Work out the finished part from the listing and answer in its coordinate system (mm). Round coordinates to 2 decimals unless told otherwise and drop trailing zeros. Write each loop counter-clockwise with the first axis right and the second up, starting at its lowest first coordinate (ties: lowest second). Pieces come first, ordered by that corner, then holes. Notation, with made-up numbers: (74, -13.5) -> (126, -13.5) arc R11 cw to (126, 5.5) -> close; hole circle Ø4 at (35.5, 53). An arc over 180 degrees is marked (long way). Answer as a JSON object with one key per item and string values. Group by question number.
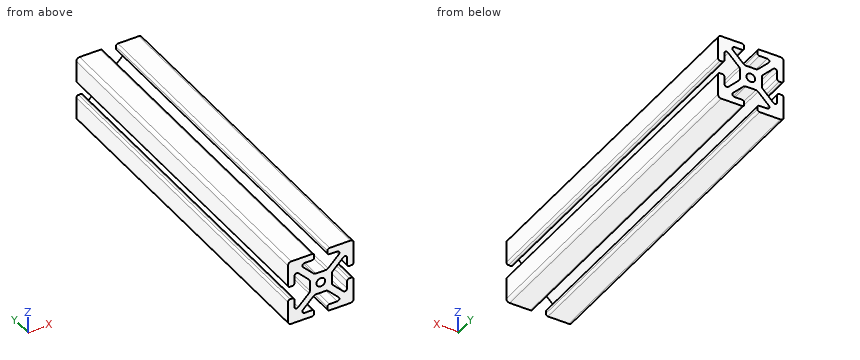
from build123d import *

# Parameters (mm, degrees)
F0_R     = 2
F1_DEPTH = 160


with BuildPart() as f1:
    # F0 (on Front) → F1 (new body)
    with BuildSketch(Plane.XZ):
        with BuildLine():
            ThreePointArc((15, 13.5), (14.56066, 14.56066), (13.5, 15))
            Line((13.5, 15), (4, 15))
            ThreePointArc((4, 15), (3.292893, 14.707107), (3, 14))
            Line((3, 14), (3, 13))
            ThreePointArc((3, 13), (3.292893, 12.292893), (4, 12))
            Line((4, 12), (7.464466, 12))
            ThreePointArc((7.464466, 12), (8.388346, 11.382683), (8.171573, 10.292893))
            Line((8.171573, 10.292893), (3.318019, 5.43934))
            ThreePointArc((3.318019, 5.43934), (2.831384, 5.114181), (2.257359, 5))
            Line((2.257359, 5), (-2.257359, 5))
            ThreePointArc((-2.257359, 5), (-2.831384, 5.114181), (-3.318019, 5.43934))
            Line((-3.318019, 5.43934), (-8.171573, 10.292893))
            ThreePointArc((-8.171573, 10.292893), (-8.388346, 11.382683), (-7.464466, 12))
            Line((-7.464466, 12), (-4, 12))
            ThreePointArc((-4, 12), (-3.292893, 12.292893), (-3, 13))
            Line((-3, 13), (-3, 14))
            ThreePointArc((-3, 14), (-3.292893, 14.707107), (-4, 15))
            Line((-4, 15), (-13.5, 15))
            ThreePointArc((-13.5, 15), (-14.56066, 14.56066), (-15, 13.5))
            Line((-15, 13.5), (-15, 4))
            ThreePointArc((-15, 4), (-14.707107, 3.292893), (-14, 3))
            Line((-14, 3), (-13, 3))
            ThreePointArc((-13, 3), (-12.292893, 3.292893), (-12, 4))
            Line((-12, 4), (-12, 7.464466))
            ThreePointArc((-12, 7.464466), (-11.382683, 8.388346), (-10.292893, 8.171573))
            Line((-10.292893, 8.171573), (-5.43934, 3.318019))
            ThreePointArc((-5.43934, 3.318019), (-5.114181, 2.831384), (-5, 2.257359))
            Line((-5, 2.257359), (-5, -2.257359))
            ThreePointArc((-5, -2.257359), (-5.114181, -2.831384), (-5.43934, -3.318019))
            Line((-5.43934, -3.318019), (-10.292893, -8.171573))
            ThreePointArc((-10.292893, -8.171573), (-11.382683, -8.388346), (-12, -7.464466))
            Line((-12, -7.464466), (-12, -4))
            ThreePointArc((-12, -4), (-12.292893, -3.292893), (-13, -3))
            Line((-13, -3), (-14, -3))
            ThreePointArc((-14, -3), (-14.707107, -3.292893), (-15, -4))
            Line((-15, -4), (-15, -13.5))
            ThreePointArc((-15, -13.5), (-14.56066, -14.56066), (-13.5, -15))
            Line((-13.5, -15), (-4, -15))
            ThreePointArc((-4, -15), (-3.292893, -14.707107), (-3, -14))
            Line((-3, -14), (-3, -13))
            ThreePointArc((-3, -13), (-3.292893, -12.292893), (-4, -12))
            Line((-4, -12), (-7.464466, -12))
            ThreePointArc((-7.464466, -12), (-8.388346, -11.382683), (-8.171573, -10.292893))
            Line((-8.171573, -10.292893), (-3.318019, -5.43934))
            ThreePointArc((-3.318019, -5.43934), (-2.831384, -5.114181), (-2.257359, -5))
            Line((-2.257359, -5), (2.257359, -5))
            ThreePointArc((2.257359, -5), (2.831384, -5.114181), (3.318019, -5.43934))
            Line((3.318019, -5.43934), (8.171573, -10.292893))
            ThreePointArc((8.171573, -10.292893), (8.388346, -11.382683), (7.464466, -12))
            Line((7.464466, -12), (4, -12))
            ThreePointArc((4, -12), (3.292893, -12.292893), (3, -13))
            Line((3, -13), (3, -14))
            ThreePointArc((3, -14), (3.292893, -14.707107), (4, -15))
            Line((4, -15), (13.5, -15))
            ThreePointArc((13.5, -15), (14.56066, -14.56066), (15, -13.5))
            Line((15, -13.5), (15, -4))
            ThreePointArc((15, -4), (14.707107, -3.292893), (14, -3))
            Line((14, -3), (13, -3))
            ThreePointArc((13, -3), (12.292893, -3.292893), (12, -4))
            Line((12, -4), (12, -7.464466))
            ThreePointArc((12, -7.464466), (11.382683, -8.388346), (10.292893, -8.171573))
            Line((10.292893, -8.171573), (5.43934, -3.318019))
            ThreePointArc((5.43934, -3.318019), (5.114181, -2.831384), (5, -2.257359))
            Line((5, -2.257359), (5, 2.257359))
            ThreePointArc((5, 2.257359), (5.114181, 2.831384), (5.43934, 3.318019))
            Line((5.43934, 3.318019), (10.292893, 8.171573))
            ThreePointArc((10.292893, 8.171573), (11.382683, 8.388346), (12, 7.464466))
            Line((12, 7.464466), (12, 4))
            ThreePointArc((12, 4), (12.292893, 3.292893), (13, 3))
            Line((13, 3), (14, 3))
            ThreePointArc((14, 3), (14.707107, 3.292893), (15, 4))
            Line((15, 4), (15, 13.5))
        make_face()
        Circle(F0_R, mode=Mode.SUBTRACT)
    extrude(amount=-F1_DEPTH)


solid = f1.part
1) A cutting plane is placed at A-A on x = 0. Determine the outline of the cut face in (y, z).
2) Straight lines are drawn through the part: L1, parallel to Z at x = 0, y = 45; L2, parallel to X at y = 98.5, z = 11; L3, parallel to Z at x = 8, y = 41.5. For each, find the intervals that lie inside material, in ascending order.
3) Each of these flat-tipped pins is pushed along its axis until it touches: P1, Ø3.5, axis at y = 67, z = 1, coming from the +X side; P2, Ø3.5, axis at y = 114, z = 0.5, coming from the -X side; P3, Ø1.5, axis at x = -3, y = 90, coming from the +Z side. Where does it stop, or does it pass through?
4) A cutting plane is placed at B-B on z = 0. Determine the outline of the cut face in (x, y), plus the area to 3 significant figures.
Established:
{
 "1": {"outline": "(0, -5) -> (160, -5) -> (160, -2) -> (0, -2) -> close; (0, 2) -> (160, 2) -> (160, 5) -> (0, 5) -> close"},
 "2": {"L1": "z = -5 to -2, 2 to 5", "L2": "x = -15 to -8.46, 8.46 to 15", "L3": "z = -15 to -11.84, -10.12 to -5.88, 5.88 to 10.12, 11.84 to 15"},
 "3": {"P1": "stops at x = 5.08", "P2": "stops at x = -5", "P3": "stops at z = 14.97"},
 "4": {"outline": "(-5, 0) -> (-2, 0) -> (-2, 160) -> (-5, 160) -> close; (2, 0) -> (5, 0) -> (5, 160) -> (2, 160) -> close", "area": "960 mm²"}
}
